Job drawing, mm, ordinate dimensions from the low corner. One solid piece. A direction names the side the tool comes from. Round coordinates to 2 decimals unless told otherwise and drop trailing zeros. Order: outer loops, then holes, each group sorted by start corner. A loop starts at its lowest first (then second) coordinate and runs counter-clockwise, first axis right, second up. Notation, with made-up numbers: (42, -25) -> (48, -25) arc R22 ccw to (48, 5) -> close; hole circle Ø8 at (37, -39). An arc over 180 degrees is marked (long way). Answer as a JSON object with one key per item and string values. Group by question number.
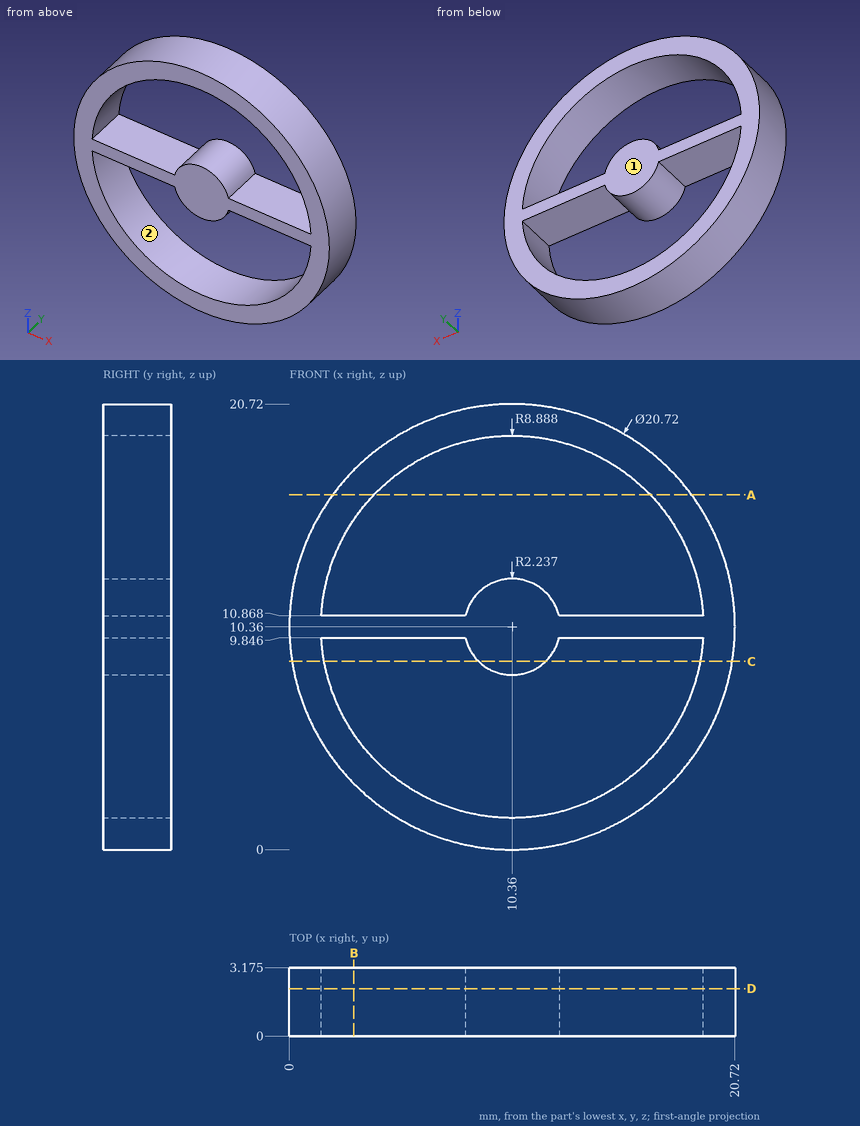
Q1. Band-saw the part on D-D (y = 2.2). List the corners of the cut face in (x, z) (1 decimal).
Q2. Band-saw the part on B-B (x = 3). List the corners of the cut face in (y, z) (1 decimal), plus the area to 3 significant figures.
Q3. Band-saw the part on C-C (z = 8.75). List the corners of the cut face in (x, y) (1 decimal).
Q4. Band-saw the part on A-A (z = 16.5). List the corners of the cut face in (x, y) (1 decimal), plus the area to 3 significant figures.
Q5. Which spindle directions (+Z, -Z, +X, -X, +Y, -Y) get a long thin tool onto all of the face, cutting with end or side? Do the marked faces 1 and 2. Say none if no direction does.
Q6. Wall check: line 1 (Z direction, x = 15.5, y = 0.7) (1 decimal); line 2 (Z direction, x = 13, y = 0.9) (1 decimal); line 3 (X direction, y = 1.4, z = 8.75) (1 decimal). Give the ranges that are in metal, low to high. Write a range as [from, to].
Q7. Drop a flat-ended pin along its axis: pin 1 Ø1.6 at (x, y) = (17.5, 1.5) entering from +Z (1 decimal). Give the stop position or say it passes through.
Completed:
{
 "1": {"outline": "circle Ø20.7 at (10.4, 10.4); hole (1.5, 9.8) arc R8.9 ccw to (19.2, 9.8) -> (12.5, 9.8) arc R2.2 cw to (8.2, 9.8) -> close; hole (1.5, 10.9) -> (8.2, 10.9) arc R2.2 cw to (12.5, 10.9) -> (19.2, 10.9) arc R8.9 ccw to start"},
 "2": {"outline": "(0, 3.1) -> (3.2, 3.1) -> (3.2, 5.4) -> (0, 5.4) -> close; (0, 9.8) -> (3.2, 9.8) -> (3.2, 10.9) -> (0, 10.9) -> close; (0, 15.3) -> (3.2, 15.3) -> (3.2, 17.7) -> (0, 17.7) -> close", "area": "17.9 mm2"},
 "3": {"outline": "(0.1, 0) -> (1.6, 0) -> (1.6, 3.2) -> (0.1, 3.2) -> close; (8.8, 0) -> (11.9, 0) -> (11.9, 3.2) -> (8.8, 3.2) -> close; (19.1, 0) -> (20.6, 0) -> (20.6, 3.2) -> (19.1, 3.2) -> close"},
 "4": {"outline": "(2, 0) -> (3.9, 0) -> (3.9, 3.2) -> (2, 3.2) -> close; (16.8, 0) -> (18.7, 0) -> (18.7, 3.2) -> (16.8, 3.2) -> close", "area": "12.2 mm2"},
 "5": {"face 1": "+Z, -Z, +X, -X, +Y", "face 2": "+Y, -Y"},
 "6": {"line 1": "[1.4, 3.1], [9.8, 10.9], [17.6, 19.4]", "line 2": "[0.3, 1.9], [9.8, 10.9], [18.8, 20.4]", "line 3": "[0.1, 1.6], [8.8, 11.9], [19.1, 20.6]"},
 "7": {"pin 1": "z = 18.6"}
}
